```python
from build123d import *

# Parameters (mm, degrees)
SALIENTE_EXTRUIR1_DEPTH = 3
CROQUIS2_R              = 1.5875
CORTAR_EXTRUIR1_DEPTH   = 20
CROQUIS3_R              = 2.38125
CORTAR_EXTRUIR2_DEPTH   = 10


with BuildPart() as part:
    # Croquis1 → Saliente-Extruir1 (new body)
    with BuildSketch(Plane(origin=(0, 0, 0), x_dir=(1, 0, 0), z_dir=(0, 1, 0))):
        with BuildLine():
            Line((10, 0), (100, 0))
            ThreePointArc((100, 0), (107.071067812, 2.928932188), (110, 10))
            Line((110, 10), (110, 240))
            ThreePointArc((110, 240), (107.071067812, 247.071067812), (100, 250))
            Line((100, 250), (10, 250))
            ThreePointArc((10, 250), (2.928932188, 247.071067812), (0, 240))
            Line((0, 240), (0, 10))
            ThreePointArc((0, 10), (2.928932188, 2.928932188), (10, 0))
        make_face()
    extrude(amount=SALIENTE_EXTRUIR1_DEPTH)

    # Croquis2 → Cortar-Extruir1 (cut)
    with BuildSketch(Plane(origin=(0, 3, 0), x_dir=(1, 0, 0), z_dir=(0, 1, 0))):
        with Locations((30, 237.3)):
            Circle(CROQUIS2_R)
        with Locations((80, 237.3)):
            Circle(CROQUIS2_R)
        with Locations((30, 12.7)):
            Circle(CROQUIS2_R)
        with Locations((80, 12.7)):
            Circle(CROQUIS2_R)
    extrude(amount=-CORTAR_EXTRUIR1_DEPTH, mode=Mode.SUBTRACT)

    # Croquis3 → Cortar-Extruir2 (cut)
    with BuildSketch(Plane(origin=(0, 3, 0), x_dir=(1, 0, 0), z_dir=(0, 1, 0))):
        with Locations((26, 60)):
            Circle(CROQUIS3_R)
        with Locations((84, 60)):
            Circle(CROQUIS3_R)
        with Locations((26, 43)):
            Circle(CROQUIS3_R)
        with Locations((84, 43)):
            Circle(CROQUIS3_R)
    extrude(amount=-CORTAR_EXTRUIR2_DEPTH, mode=Mode.SUBTRACT)


solid = part.part
```
CAD build for the part. Positions are in the model's coordinates, mm. Round coordinates to 2 decimals unless told otherwise and drop trailing zeros. Write each loop counter-clockwise with the first axis right and the second up, starting at its lowest first coordinate (ties: lowest second). Pieces come first, ordered by that corner, then holes. Notation, with made-up numbers: (-3, 54) - (2, 54) arc R30 ccw to (2, 82) - close; hole circle Ø5 at (34.25, 40). An arc over 180 degrees is marked (long way). Return JSON: item names as keys, results as strings. Group by question number.
Item 1: Band-saw the part on A-A on x = 26. List the corners of the cut face in (y, z).
Item 2: Flat gauge pins, fed straight in: pin 1 Ø1.5 at (x, z) = (37, -103) entering from -Y; pin 2 Ø1.9 at (x, z) = (80, -237.3) entering from +Y. Where does each tip first touch, or does it go through?
Item 3: Mould opens along Z. For faces 1 (the face through (54, 0, -127)), 2 (the face through (82.11, 1.52, -58.55)), 3 (the face through (2.85, 1.48, -3.01)) say: +Z half, -Z half, draft (parallel to the pull), parting line (faces both ways), or undercut.
Item 4: Probe probe 1 along X at (y, z) = (1.3, -237.3); probe 2 along Z at (x, y) = (26.5, 0.95); probe 3 along Z at (x, y) = (30, 2). List the from-to ranges inside material, lowest first.
Resolved:
{
 "1": {"outline": "(0, -250) - (3, -250) - (3, -62.38) - (0, -62.38) - close; (0, -57.62) - (3, -57.62) - (3, -45.38) - (0, -45.38) - close; (0, -40.62) - (3, -40.62) - (3, 0) - (0, 0) - close"},
 "2": {"pin 1": "stops at y = 0", "pin 2": "passes through"},
 "3": {"face 1": "draft", "face 2": "undercut", "face 3": "+Z half"},
 "4": {"probe 1": "x = 0 to 28.41, 31.59 to 78.41, 81.59 to 110", "probe 2": "z = -250 to -62.33, -57.67 to -45.33, -40.67 to 0", "probe 3": "z = -250 to -238.89, -235.71 to -14.29, -11.11 to 0"}
}
